Verification items for the finished model (mm, model axes). Face numbers are marked on the shaded views. A direction names the side the tool comes from. Give positions to 0.01 mm unless a question says otherwise; leave off trailing zeros. Order: outer loops, then holes, each group sorted by start corner. A loop starts at its lowest first (then second) coordinate and runs counter-clockwise, first axis right, second up. Notation, with made-up numbers: (32.5, 32.5) - (77.5, 32.5) arc R7 ccw to (77.5, 40.5) - close; hole circle Ø5 at (-24, -38). An arc over 180 degrees is marked (long way). Answer as a JSON object with one key per item and string values. Group by question number.
(1) Access from +Z, -Z, +X, -X, +Y, -Y to the whole of each face (thin tool, end or side, straight path). Record for the marked faces 4, 5, 6 and 7.
(2) Section check B-B (z = -17). Record the boundary of the cut face in (x, y), then the cut area to 3 significant figures.
(3) Thickness scan on line 1 (Z direction, x = -219, y = -109.5); line 2 (X direction, y = -68, z = 103.5); line 3 (X direction, y = 45, z = 123). Record the ranges inside material, lowest first.
(4) Section check D-D (y = -22.5). Record the boundary of the cut face in (x, z).
(5) Mould release check, pull along Z, two halves, no side actions. Record for the marked faces 1, 2 and 3: +Z half, -Z half, draft (parallel to the pull), parting line (faces both ways), or undercut.
(6) Depth check by flat-ended pin: pin 1 Ø1.4 at (x, y) = (62, 44.5) entering from +Z; pin 2 Ø1.6 at (x, y) = (-235, 44.5) entering from +Z; pin 3 Ø12 at (y, z) = (-14, 85.5) entering from +X. Enter the tip coordinate at first touch or a pass-through.
(7) Section check A-A (y = -95). Record the boundary of the cut face in (x, z).
(8) Section check C-C (x = -49.5). Record the boundary of the cut face in (y, z).
```python
from build123d import *

# Parameters (mm, degrees)
SKETCH1_W                       = 280
SKETCH1_H                       = 205
BASE_FLANGE1_DEPTH              = 2
EDGE_FLANGE1_STRIP_W            = 12
EDGE_FLANGE1_STRIP_H            = 2
EDGE_FLANGE1_STRIP_CUT_DEPTH    = 205
EDGE_FLANGE1_DEPTH              = 205
EDGE_FLANGE2_STRIP_W            = 12
EDGE_FLANGE2_STRIP_H            = 2
EDGE_FLANGE2_STRIP_CUT_DEPTH    = 205
EDGE_FLANGE2_DEPTH              = 205
EDGE_FLANGE3_STRIP_W            = 12
EDGE_FLANGE3_STRIP_H            = 2
EDGE_FLANGE3_STRIP_CUT_DEPTH    = 205
EDGE_FLANGE3_DEPTH              = 205
SKETCH15_W                      = 240
SKETCH15_H                      = 140
CUT_EXTRUDE1_DEPTH              = 10
SKETCH16_R                      = 17
CUT_EXTRUDE2_DEPTH              = 10
EDGE_FLANGE11_STRIP_W           = 9.4732
EDGE_FLANGE11_STRIP_H           = 2
EDGE_FLANGE11_STRIP_CUT_DEPTH   = 276
EDGE_FLANGE11_STRIP_2_W         = 9.4732
EDGE_FLANGE11_STRIP_2_H         = 2
EDGE_FLANGE11_STRIP_CUT_2_DEPTH = 102
EDGE_FLANGE11_STRIP_3_W         = 9.4732
EDGE_FLANGE11_STRIP_3_H         = 2
EDGE_FLANGE11_STRIP_CUT_3_DEPTH = 272
EDGE_FLANGE11_STRIP_4_W         = 9.4732
EDGE_FLANGE11_STRIP_4_H         = 2
EDGE_FLANGE11_STRIP_CUT_4_DEPTH = 103.9
EDGE_FLANGE11_DEPTH             = 276
EDGE_FLANGE11_BEND_DEPTH        = 102
EDGE_FLANGE11_BEND_2_DEPTH      = 272
EDGE_FLANGE11_BEND_3_DEPTH      = 103.9
SKETCH55_R                      = 4
CUT_EXTRUDE3_DEPTH              = 10


# Sheet-metal steps are written as plain solids
with BuildPart() as part:
    # Sketch1 → Base-Flange1 (new body)
    with BuildSketch(Plane.XY):
        with Locations((-95.977777778, -56.488888889)):
            Rectangle(SKETCH1_W, SKETCH1_H)
    extrude(amount=-BASE_FLANGE1_DEPTH)

    # Edge-Flange1 strip (across the edge) → Edge-Flange1 strip cut (cut)
    with BuildSketch(Plane(origin=(-235.977777778, 46.011111111, 0), x_dir=(1, 0, 0), z_dir=(0, -1, 0))):
        with Locations((-2, -1)):
            Rectangle(EDGE_FLANGE1_STRIP_W, EDGE_FLANGE1_STRIP_H)
    extrude(amount=EDGE_FLANGE1_STRIP_CUT_DEPTH, mode=Mode.SUBTRACT)

    # Edge-Flange1 section (across the edge) → Edge-Flange1 (add)
    with BuildSketch(Plane(origin=(-235.977777778, 46.011111111, 0), x_dir=(1, 0, 0), z_dir=(0, -1, 0))):
        with BuildLine():
            Line((0, 2), (0, 108))
            Line((0, 108), (2, 108))
            Line((2, 108), (2, 2))
            ThreePointArc((2, 2), (2.585786438, 0.585786438), (4, 0))
            Line((4, 0), (4, -2))
            ThreePointArc((4, -2), (1.171572875, -0.828427125), (0, 2))
        make_face()
    extrude(amount=EDGE_FLANGE1_DEPTH)

    # Edge-Flange2 strip (across the edge) → Edge-Flange2 strip cut (cut)
    with BuildSketch(Plane(origin=(-233.977777778, 46.011111111, 108), x_dir=(0, 0, -1), z_dir=(0, -1, 0))):
        with Locations((-2, -1)):
            Rectangle(EDGE_FLANGE2_STRIP_W, EDGE_FLANGE2_STRIP_H)
    extrude(amount=EDGE_FLANGE2_STRIP_CUT_DEPTH, mode=Mode.SUBTRACT)

    # Edge-Flange2 section (across the edge) → Edge-Flange2 (add)
    with BuildSketch(Plane(origin=(-233.977777778, 46.011111111, 108), x_dir=(0, 0, -1), z_dir=(0, -1, 0))):
        with BuildLine():
            Line((0, 2), (0, 278))
            Line((0, 278), (2, 278))
            Line((2, 278), (2, 2))
            ThreePointArc((2, 2), (2.585786438, 0.585786438), (4, 0))
            Line((4, 0), (4, -2))
            ThreePointArc((4, -2), (1.171572875, -0.828427125), (0, 2))
        make_face()
    extrude(amount=EDGE_FLANGE2_DEPTH)

    # Edge-Flange3 strip (across the edge) → Edge-Flange3 strip cut (cut)
    with BuildSketch(Plane(origin=(44.022222222, 46.011111111, 106), x_dir=(-1, 0, 0), z_dir=(0, -1, 0))):
        with Locations((-2, -1)):
            Rectangle(EDGE_FLANGE3_STRIP_W, EDGE_FLANGE3_STRIP_H)
    extrude(amount=EDGE_FLANGE3_STRIP_CUT_DEPTH, mode=Mode.SUBTRACT)

    # Edge-Flange3 section (across the edge) → Edge-Flange3 (add)
    with BuildSketch(Plane(origin=(44.022222222, 46.011111111, 106), x_dir=(-1, 0, 0), z_dir=(0, -1, 0))):
        with BuildLine():
            Line((0, 2), (0, 105.9))
            Line((0, 105.9), (2, 105.9))
            Line((2, 105.9), (2, 2))
            ThreePointArc((2, 2), (2.585786438, 0.585786438), (4, 0))
            Line((4, 0), (4, -2))
            ThreePointArc((4, -2), (1.171572875, -0.828427125), (0, 2))
        make_face()
    extrude(amount=EDGE_FLANGE3_DEPTH)

    # Sketch15 → Cut-Extrude1 (cut)
    with BuildSketch(Plane.XY.offset(108)):
        with Locations((-95.977777778, -56.488888889)):
            Rectangle(SKETCH15_W, SKETCH15_H)
    extrude(amount=-CUT_EXTRUDE1_DEPTH, mode=Mode.SUBTRACT)

    # Sketch16 → Cut-Extrude2 (cut)
    with BuildSketch(Plane(origin=(0, 0, -2), x_dir=(-1, 0, 0), z_dir=(0, 0, -1))):
        with Locations((97.977777778, -10.988888889)):
            Circle(SKETCH16_R)
    extrude(amount=-CUT_EXTRUDE2_DEPTH, mode=Mode.SUBTRACT)

    # Edge-Flange11 strip (across the edge) → Edge-Flange11 strip cut (cut)
    with BuildSketch(Plane(origin=(-231.977777778, 46.011111111, -2), x_dir=(0, -1, 0), z_dir=(1, 0, 0))):
        with Locations((-2, -1)):
            Rectangle(EDGE_FLANGE11_STRIP_W, EDGE_FLANGE11_STRIP_H)
    extrude(amount=EDGE_FLANGE11_STRIP_CUT_DEPTH, mode=Mode.SUBTRACT)

    # Edge-Flange11 strip 2 (across the edge) → Edge-Flange11 strip cut 2 (cut)
    with BuildSketch(Plane(origin=(-235.977777778, 46.011111111, 104), x_dir=(0, -1, 0), z_dir=(0, 0, -1))):
        with Locations((-2, -1)):
            Rectangle(EDGE_FLANGE11_STRIP_2_W, EDGE_FLANGE11_STRIP_2_H)
    extrude(amount=EDGE_FLANGE11_STRIP_CUT_2_DEPTH, mode=Mode.SUBTRACT)

    # Edge-Flange11 strip 3 (across the edge) → Edge-Flange11 strip cut 3 (cut)
    with BuildSketch(Plane(origin=(40.022222222, 46.011111111, 108), x_dir=(0, -1, 0), z_dir=(-1, 0, 0))):
        with Locations((-2, -1)):
            Rectangle(EDGE_FLANGE11_STRIP_3_W, EDGE_FLANGE11_STRIP_3_H)
    extrude(amount=EDGE_FLANGE11_STRIP_CUT_3_DEPTH, mode=Mode.SUBTRACT)

    # Edge-Flange11 strip 4 (across the edge) → Edge-Flange11 strip cut 4 (cut)
    with BuildSketch(Plane(origin=(44.022222222, 46.011111111, 0.1), x_dir=(0, -1, 0), z_dir=(0, 0, 1))):
        with Locations((-2, -1)):
            Rectangle(EDGE_FLANGE11_STRIP_4_W, EDGE_FLANGE11_STRIP_4_H)
    extrude(amount=EDGE_FLANGE11_STRIP_CUT_4_DEPTH, mode=Mode.SUBTRACT)

    # Edge-Flange11 section (across the edge) → Edge-Flange11 (add)
    with BuildSketch(Plane(origin=(-231.977777778, 46.011111111, -2), x_dir=(0, -1, 0), z_dir=(1, 0, 0))):
        with BuildLine():
            Line((0, 0.7366), (0, 30))
            Line((0, 30), (2, 30))
            Line((2, 30), (2, 0.7366))
            ThreePointArc((2, 0.7366), (2.215745145, 0.215745145), (2.7366, 0))
            Line((2.7366, 0), (2.7366, -2))
            ThreePointArc((2.7366, -2), (0.801531583, -1.198468417), (0, 0.7366))
        make_face()
    extrude(amount=EDGE_FLANGE11_DEPTH)

    # Edge-Flange11 section 2 (across the edge) → Edge-Flange11 bend (add)
    with BuildSketch(Plane(origin=(-235.977777778, 46.011111111, 104), x_dir=(0, -1, 0), z_dir=(0, 0, -1))):
        with BuildLine():
            Line((0, 0.7366), (0, 30))
            Line((0, 30), (2, 30))
            Line((2, 30), (2, 0.7366))
            ThreePointArc((2, 0.7366), (2.215745145, 0.215745145), (2.7366, 0))
            Line((2.7366, 0), (2.7366, -2))
            ThreePointArc((2.7366, -2), (0.801531583, -1.198468417), (0, 0.7366))
        make_face()
    extrude(amount=EDGE_FLANGE11_BEND_DEPTH)

    # Edge-Flange11 section 3 (across the edge) → Edge-Flange11 bend 2 (add)
    with BuildSketch(Plane(origin=(40.022222222, 46.011111111, 108), x_dir=(0, -1, 0), z_dir=(-1, 0, 0))):
        with BuildLine():
            Line((0, 0.7366), (0, 30))
            Line((0, 30), (2, 30))
            Line((2, 30), (2, 0.7366))
            ThreePointArc((2, 0.7366), (2.215745145, 0.215745145), (2.7366, 0))
            Line((2.7366, 0), (2.7366, -2))
            ThreePointArc((2.7366, -2), (0.801531583, -1.198468417), (0, 0.7366))
        make_face()
    extrude(amount=EDGE_FLANGE11_BEND_2_DEPTH)

    # Edge-Flange11 section 4 (across the edge) → Edge-Flange11 bend 3 (add)
    with BuildSketch(Plane(origin=(44.022222222, 46.011111111, 0.1), x_dir=(0, -1, 0), z_dir=(0, 0, 1))):
        with BuildLine():
            Line((0, 0.7366), (0, 30))
            Line((0, 30), (2, 30))
            Line((2, 30), (2, 0.7366))
            ThreePointArc((2, 0.7366), (2.215745145, 0.215745145), (2.7366, 0))
            Line((2.7366, 0), (2.7366, -2))
            ThreePointArc((2.7366, -2), (0.801531583, -1.198468417), (0, 0.7366))
        make_face()
    extrude(amount=EDGE_FLANGE11_BEND_3_DEPTH)

    # Sketch55 → Cut-Extrude3 (cut)
    with BuildSketch(Plane.XZ.offset(-44.011111111)):
        with Locations(Location((-95.977777778, -17, 0), (0, 0, 270))):
            Circle(SKETCH55_R)
        with Locations(Location((-95.977777778, 123, 0), (0, 0, 270))):
            Circle(SKETCH55_R)
    extrude(amount=-CUT_EXTRUDE3_DEPTH, mode=Mode.SUBTRACT)


solid = part.part
```
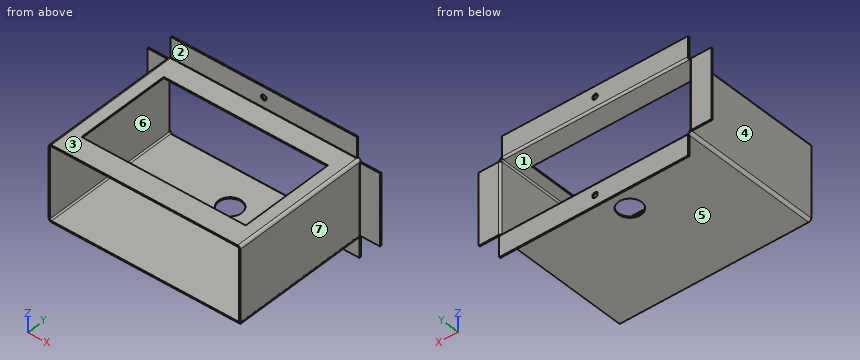
Solutions:
{
 "1": {"face 4": "+Z, -Z, -X, -Y", "face 5": "-Z, +X, -X, -Y", "face 6": "+Y, -Y", "face 7": "+Z, -Z, +X, -Y"},
 "2": {"outline": "(-231.98, 44.01) - (-99.98, 44.01) - (-99.98, 46.01) - (-231.98, 46.01) - close; (-91.98, 44.01) - (44.02, 44.01) - (44.02, 46.01) - (-91.98, 46.01) - close", "area": "536 mm2"},
 "3": {"line 1": "z = -2 to 0, 106 to 108", "line 2": "x = -235.98 to -233.98, 42.02 to 44.02", "line 3": "x = -231.98 to -99.98, -91.98 to 40.02"},
 "4": {"outline": "(-235.98, 2) arc R4 ccw to (-231.98, -2) - (-110.49, -2) - (-110.49, 0) - (-231.98, 0) arc R2 cw to (-233.98, 2) - (-233.98, 104) arc R2 cw to (-231.98, 106) - (-215.98, 106) - (-215.98, 108) - (-231.98, 108) arc R4 ccw to (-235.98, 104) - close; (-85.47, -2) - (44.02, -2) - (44.02, 0) - (-85.47, 0) - close; (24.02, 106) - (40.02, 106) arc R2 cw to (42.02, 104) - (42.02, 0.1) - (44.02, 0.1) - (44.02, 104) arc R4 ccw to (40.02, 108) - (24.02, 108) - close"},
 "5": {"face 1": "undercut", "face 2": "draft", "face 3": "+Z half"},
 "6": {"pin 1": "stops at z = 104", "pin 2": "stops at z = 107.33", "pin 3": "stops at x = 44.02"},
 "7": {"outline": "(-235.98, 2) arc R4 ccw to (-231.98, -2) - (44.02, -2) - (44.02, 0) - (-231.98, 0) arc R2 cw to (-233.98, 2) - (-233.98, 104) arc R2 cw to (-231.98, 106) - (-215.98, 106) - (-215.98, 108) - (-231.98, 108) arc R4 ccw to (-235.98, 104) - close; (24.02, 106) - (40.02, 106) arc R2 cw to (42.02, 104) - (42.02, 0.1) - (44.02, 0.1) - (44.02, 104) arc R4 ccw to (40.02, 108) - (24.02, 108) - close"},
 "8": {"outline": "(-158.99, -2) - (43.27, -2) arc R0.74 cw to (44.01, -2.74) - (44.01, -32) - (46.01, -32) - (46.01, -2.74) arc R2.74 ccw to (43.27, 0) - (-158.99, 0) - close; (-158.99, 106) - (-126.49, 106) - (-126.49, 108) - (-158.99, 108) - close; (13.51, 106) - (43.27, 106) arc R2.74 ccw to (46.01, 108.74) - (46.01, 138) - (44.01, 138) - (44.01, 108.74) arc R0.74 cw to (43.27, 108) - (13.51, 108) - close"}
}
